```python
from build123d import *

# Parameters (mm, degrees)
F1_DEPTH = 2.38125
F2_R     = 2.38125
F3_DEPTH = 25.4
F5_DEPTH = 25.4


with BuildPart() as f1:
    # F0 (on Front) → F1 (new body)
    with BuildSketch(Plane.XZ):
        with BuildLine():
            Line((60.325, 19.05), (7.9375, 19.05))
            ThreePointArc((7.9375, 19.05), (2.32484, 16.72516), (0, 11.1125))
            Line((0, 11.1125), (0, 0))
            Line((0, 0), (9.525, 0))
            Line((9.525, 0), (12.144122, 7.72185))
            ThreePointArc((12.144122, 7.72185), (13.224173, 12.410645), (17.480062, 14.655354))
            Line((17.480062, 14.655354), (60.325, 17.05))
            Line((60.325, 17.05), (60.325, 19.05))
        make_face()
    extrude(amount=F1_DEPTH)

    # F2 (on face) → F3 (cut)
    with BuildSketch(Plane.XZ.offset(2.38125)):
        with Locations((7.9375, 11.1125)):
            Circle(F2_R)
    extrude(amount=-F3_DEPTH, mode=Mode.SUBTRACT)

    # F4 (on face) → F5 (cut)
    with BuildSketch(Plane.XY.offset(19.05)):
        Polygon((60.325, 0), (45.24375, 0), (60.325, -0.79375), align=None)
        Polygon((60.325, -2.38125), (60.325, -1.5875), (45.24375, -2.38125), align=None)
    extrude(amount=-F5_DEPTH, mode=Mode.SUBTRACT)


solid = f1.part
```
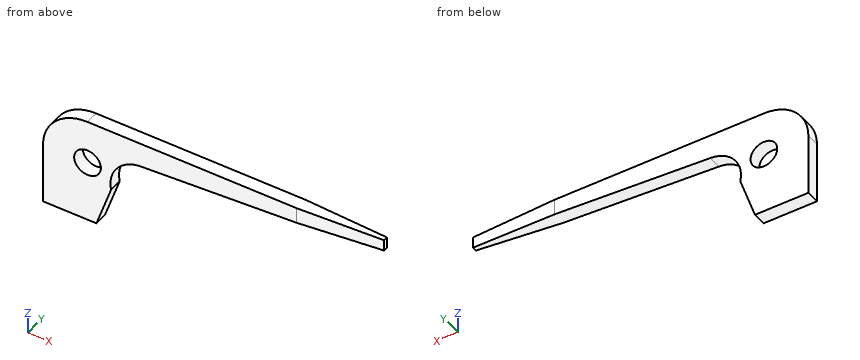
Here's how the part is built. I have some questions about the finished solid (model axes, mm). Coordinates: 2 decimals unless noted, no trailing zeros. Order: outer loops, then holes, each group sorted by start corner. A loop starts at its lowest first (then second) coordinate and runs counter-clockwise, first axis right, second up. Notation, with made-up numbers: M -6,-36 L 2,-36 A15 cw 2,-29 Z; hole C -27,80 d7. An arc over 180 degrees is marked long. Answer as a JSON object with one key per item and string values. Group by question number.
(1) Suppose I cut it at A-A, the plane x = 8.5. Please give me the cut outline in (y, z), then the cut area to 3 significant figures.
(2) Suppose I cut it at B-B, the plane z = 9.25. Please give me the cut outline in (x, y).
(3) I need wall thicknesses on probe 1 along Z at (x, y) = (7, -0.4); probe 2 along X at (y, z) = (-0.7, 9.5); probe 3 along Z at (x, y) = (38, -0.4). Which ranges of each line are inside material? Lowest first, please.
(4) Suppose I cut it at D-D, the plane z = 17.75. Please give me the cut outline in (x, y) (1 decimal).
(5) For pin 1 (5.5 mm diameter, centred on x = 7.94, z = 11.11, fed in from +Y); pin 2 (1 mm diameter, centred on y = -1.5, z = 16.5, fed in from -X), each with a flat end and sliding along its axis, tell me the tip position at first contact or that it passes through.
Values found:
{
 "1": {"outline": "M -2.38,0 L 0,0 L 0,8.8 L -2.38,8.8 Z; M -2.38,13.43 L 0,13.43 L 0,19.05 L -2.38,19.05 Z", "area": "34.3 mm^2"},
 "2": {"outline": "M 0,-2.38 L 6.45,-2.38 L 6.45,0 L 0,0 Z; M 9.42,-2.38 L 12.04,-2.38 L 12.04,0 L 9.42,0 Z"},
 "3": {"probe 1": "z = 0 to 8.92, 13.3 to 18.99", "probe 2": "x = 0 to 6.19, 9.69 to 12.06", "probe 3": "z = 15.8 to 19.05"},
 "4": {"outline": "M 3.6,-2.4 L 45.2,-2.4 L 60.3,-1.6 L 60.3,-0.8 L 45.2,0 L 3.6,0 Z"},
 "5": {"pin 1": "stops at y = 0", "pin 2": "stops at x = 1.68"}
}
